```python
from build123d import *

# Parameters (mm, degrees)
SKETCH2_R          = 3
CUT_EXTRUDE1_DEPTH = 15
ECHELLE1_SCALE     = 0.5


with BuildPart() as part:
    # Sketch1 → Revolve1 (revolve)
    with BuildSketch(Plane.XY, mode=Mode.PRIVATE) as revolve1_sk:
        Polygon((-11.2, 18.1), (-1, 18.1), (-1, 9), (-12.2, 9), (-12.2, 0), (12.2, 0), (12.2, 9), (1, 9), (1, 18.1), (11.2, 18.1), (11.2, 36.4), (-11.2, 36.4), align=None)
    revolve(revolve1_sk.sketch.rotate(Axis((0, 0, 0), (1, 0, 0)), 90), axis=Axis((0, 0, 0), (1, 0, 0)))

    # Sketch2 → Cut-Extrude1 (cut)
    with BuildSketch(Plane(origin=(12.2, 0, 0), x_dir=(0, 0, -1), z_dir=(1, 0, 0))):
        Circle(SKETCH2_R)
    extrude(amount=-CUT_EXTRUDE1_DEPTH, mode=Mode.SUBTRACT)


with BuildPart() as part_1:
    # Echelle1: scaled about (-0.025714015, 0, 0)
    add(part.part.scale(ECHELLE1_SCALE).moved(Location((-0.012857007, 0, 0))))


solid = part_1.part
```
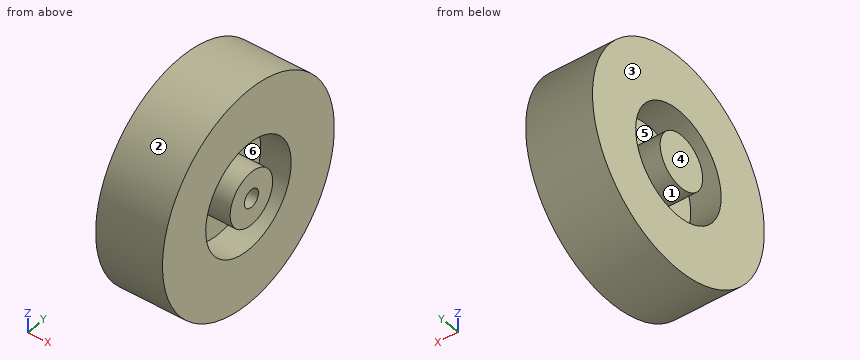
The model under review builds one solid part; all positions refer to its coordinate system, in mm. Face numbers are marked on the shaded views. A direction names the side the tool comes from. Give positions to 0.01 mm unless a question says otherwise; leave off trailing zeros. Write each loop counter-clockwise with the first axis right and the second up, starting at its lowest first coordinate (ties: lowest second). Pieces come first, ordered by that corner, then holes. Notation, with made-up numbers: M 82.5,42 L 105.5,42 A22 cw 105.5,66 Z; hole C -18.75,2.25 d4. An arc over 180 degrees is marked long. Write item = value, one per line. Start each with the question number.
Q1. We need section A-A (x = -2.5). State the section outline as (y, z) points, plus the area to 3 significant figures.
Q2. For line 1 (Y direction, x = 2.6, z = 0); line 2 (Y direction, x = -4.45, z = 0); line 3 (Z direction, x = 5.25, y = 1), list the stretches that pass through material, from the lowest coordinate up.
Q3. Mouldability with a two-part tool opening along Z and no side actions: class the marked faces 1, 2 and 3 as released by +Z, released by -Z, zero draft, split by the parting line, or undercut.
Q4. Machinability: for the marked faces 4, 5 and 6, which of the approach directions +Z, -Z, +X, -X, +Y, -Y give a long, thin tool a straight path to every point of the face, cutting with its end or side? Answer none if there is none.
Q5. We need section B-B (y = 0). State the section outline as (x, z) points.
Q6. We need section D-D (y = -14). State the section outline as (x, z) points.
Q7. Clearance check with flat-ended pins moving along their axes: pin 1 (3 mm diameter, centred on x = 1.5, y = -3.5, fed in from -Z); pin 2 (1.5 mm diameter, centred on x = -1.5, y = 12.5, fed in from +Z); pin 3 (1 mm diameter, centred on x = -4, y = 4, fed in from +Z). State where each tip first meets the part, or that it passes through.
Result set:
q1.outline = C 0,0 d36.4; C 0,0 d9; hole C 0,0 d18.1
q1.area = 847 mm2
q2.line_1 = -18.2 to -9.05, -4.5 to -1.5, 1.5 to 4.5, 9.05 to 18.2
q2.line_2 = -18.2 to -9.05, -4.5 to 4.5, 9.05 to 18.2
q2.line_3 = -18.17 to -8.99, -4.39 to -1.12, 1.12 to 4.39, 8.99 to 18.17
q3.face_1 = undercut
q3.face_2 = split by the parting line
q3.face_3 = zero draft
q4.face_4 = +Z, -Z, -X, +Y, -Y
q4.face_5 = -X
q4.face_6 = +X
q5.outline = M -6.11,-4.5 L -0.51,-4.5 L -0.51,-9.05 L -5.61,-9.05 L -5.61,-18.2 L 5.59,-18.2 L 5.59,-9.05 L 0.49,-9.05 L 0.49,-4.5 L 6.09,-4.5 L 6.09,-1.5 L -1.41,-1.5 L -1.41,1.5 L 6.09,1.5 L 6.09,4.5 L 0.49,4.5 L 0.49,9.05 L 5.59,9.05 L 5.59,18.2 L -5.61,18.2 L -5.61,9.05 L -0.51,9.05 L -0.51,4.5 L -6.11,4.5 Z
q6.outline = M -5.61,-11.63 L 5.59,-11.63 L 5.59,11.63 L -5.61,11.63 Z
q7.pin_1 = -18.09
q7.pin_2 = 13.9
q7.pin_3 = 17.86
